from build123d import *

# Parameters (mm, degrees)
FILLET_1_R          = 0.3
CUT_EXTRUDE_1_DEPTH = 2.4
CHAMFER_1_SIZE      = 0.2


with BuildPart() as part:
    # 草图1 → 旋转1 (revolve)
    with BuildSketch(Plane(origin=(0, 0, 0), x_dir=(0, 0, -1), z_dir=(1, 0, 0))):
        Polygon((0, 0), (0, 1.5), (-6, 1.5), (-6, 2), (-16, 2), (-16, 3.5), (-19.5, 3.5), (-19.5, 0), align=None)
    revolve(axis=Axis((0, 0, 0), (0, 0, 1)))

    # 圆角1
    fillet_1_edges = [part.edges().sort_by_distance(p)[0] for p in [
        (0, -3.5, 19.5),
        (0, -3.5, 16),
    ]]
    fillet(fillet_1_edges, radius=FILLET_1_R)

    # 草图2 → 切除-拉伸1 (cut)
    with BuildSketch(Plane.XY.offset(19.5)):
        Polygon((1.732050808, 0), (0.866025404, 1.5), (-0.866025404, 1.5), (-1.732050808, 0), (-0.866025404, -1.5), (0.866025404, -1.5), align=None)
    extrude(amount=-CUT_EXTRUDE_1_DEPTH, mode=Mode.SUBTRACT)

    # 倒角1
    chamfer_1_edges = [part.edges().sort_by_distance(p)[0] for p in [
        (0, -2, 6),
    ]]
    chamfer(chamfer_1_edges, length=CHAMFER_1_SIZE)


solid = part.part
For this review, take the finished solid that the model builds, in its own axes (mm). A direction names the side the tool comes from. Give positions to 0.01 mm unless a question says otherwise; leave off trailing zeros. Write each loop counter-clockwise with the first axis right and the second up, starting at its lowest first coordinate (ties: lowest second). Pieces come first, ordered by that corner, then holes. Notation, with made-up numbers: (-36, 14.5) -> (17, 14.5) arc R16 cw to (17, 23.5) -> close; hole circle Ø7 at (42.5, -28). An arc over 180 degrees is marked (long way). Use CSV: the item, a comma, the result in double quotes.
Q1. Tool access review of faces 1 (the face through (-1.305, -0.74, 18.317)), 2 (the face through (1, -2, 16)), 3 (the face through (0, 0, 0)): name each direction out of +Z, -Z, +X, -X, +Y, -Y from which nothing blocks a thin tool from reaching the whole face with its end or side.
Conclusion:
face 1,"+Z"
face 2,"-Z"
face 3,"-Z, +X, -X, +Y, -Y"
Q2. To check wall thickness, follow probe 1 along Z at (x, y) = (-3, 1.25); probe 2 along X at (y, z) = (-3, 18.5); probe 3 along Z at (x, y) = (1.25, 0). State the ranges of each line that lie inside material, in increasing order. Write a range as [from, to].
Conclusion:
probe 1,"[16, 19.5]"
probe 2,"[-1.8, 1.8]"
probe 3,"[0, 17.1]"
Q3. Mouldability with a two-part tool opening along X and no side actions: class faces 4 (the face through (-1.5, -0.8, 19.5)), 5 (the face through (-1.293, 0.76, 18.317)), 6 (the face through (-0.07, -1.5, 3.04)) as pulls with the +X half, pulls with the -X half, needs draft (parallel to the pull), parting line crosses it, or undercut.
Conclusion:
face 4,"needs draft"
face 5,"undercut"
face 6,"parting line crosses it"
Q4. For P1, Ø2, axis at y = -1, z = 13.5, coming from the +X side; P2, Ø0.9, axis at x = 0.5, y = -0.5, coming from the +Z side; P3, Ø1.5, axis at x = 2, z = 7, coming from the +Y side, all flat-tipped, find the tip position at first contact; note any pin that passes through.
Conclusion:
P1,"x = 2"
P2,"z = 17.1"
P3,"y = 1.56"
Q5. Take a section at A-A, the plane x = 0. Write out the cut boundary in (y, z), then the cut area to 3 significant figures.
Conclusion:
outline,"(-3.5, 16.3) arc R0.3 ccw to (-3.2, 16) -> (-2, 16) -> (-2, 6.2) -> (-1.8, 6) -> (-1.5, 6) -> (-1.5, 0) -> (1.5, 0) -> (1.5, 6) -> (1.8, 6) -> (2, 6.2) -> (2, 16) -> (3.2, 16) arc R0.3 ccw to (3.5, 16.3) -> (3.5, 19.2) arc R0.3 ccw to (3.2, 19.5) -> (1.5, 19.5) -> (1.5, 17.1) -> (-1.5, 17.1) -> (-1.5, 19.5) -> (-3.2, 19.5) arc R0.3 ccw to (-3.5, 19.2) -> close"
area,"75.2 mm2"
Q6. Take a section at B-B, the plane z = 14.25. Write out the cut boundary in (x, y), then the cut area to 3 significant figures.
Conclusion:
outline,"circle Ø4 at (0, 0)"
area,"12.6 mm2"
Q7. Take a section at C-C, the plane z = 1.75. Write out the cut boundary in (x, y), then the cut area to 3 significant figures.
Conclusion:
outline,"circle Ø3 at (0, 0)"
area,"7.07 mm2"
